Design review of the part built by this model. Coordinates are the model's own, in mm. Face numbers are marked on the shaded views. A direction names the side the tool comes from. Round coordinates to 2 decimals unless told otherwise and drop trailing zeros. Loops run counter-clockwise (first coordinate to the right, second up) from the corner with the lowest first, then second, coordinate; pieces in that order, holes last. Notation, with made-up numbers: (64, -17) -> (85, -17) arc R24 ccw to (85, 1) -> close; hole circle Ø7 at (74, -34). An arc over 180 degrees is marked (long way). Use a Markdown table: item, result. Add a question column.
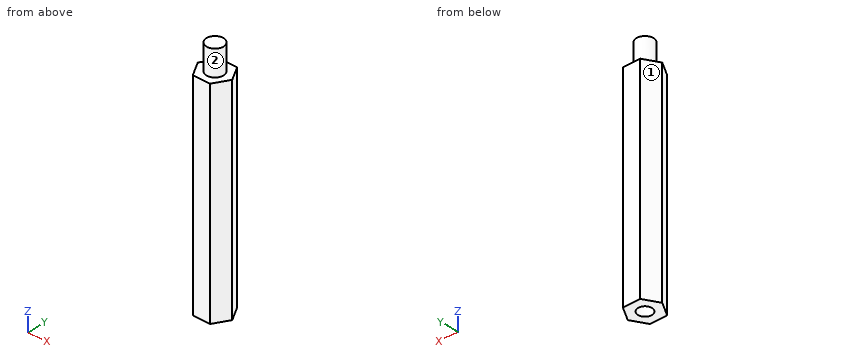
from build123d import *

# Parameters (mm, degrees)
EXTRUDE_1_DEPTH = 50
SKETCH_2_R      = 2
EXTRUDE_2_DEPTH = 6
M4X0_7_1_D      = 3.3
M4X0_7_1_DEPTH  = 10.5
M4X0_7_1_TIP    = 0.991420021


with BuildPart() as part:
    # 草圖1 → 填料-伸長1 (new body)
    with BuildSketch(Plane.XY):
        Polygon((4.041451884, 0), (2.020725942, 3.5), (-2.020725942, 3.5), (-4.041451884, 0), (-2.020725942, -3.5), (2.020725942, -3.5), align=None)
    extrude(amount=EXTRUDE_1_DEPTH)

    # 草圖2 → 填料-伸長2 (add)
    with BuildSketch(Plane.XY.offset(50)):
        Circle(SKETCH_2_R)
    extrude(amount=EXTRUDE_2_DEPTH)

    # M4x0.7 螺紋孔1
    with Locations(Plane(origin=(0, 0, 0), x_dir=(-1, 0, 0), z_dir=(0, 0, -1))):
        with Locations((0, 0)):
            Hole(M4X0_7_1_D / 2, depth=M4X0_7_1_DEPTH)
            with Locations((0, 0, -(M4X0_7_1_DEPTH + M4X0_7_1_TIP / 2))):  # 118° drill point
                Cone(0, M4X0_7_1_D / 2, M4X0_7_1_TIP, mode=Mode.SUBTRACT)


solid = part.part
1. Consider section A-A on z = 39. State the section outline as (x, y) points.
2. Insertion check: P1, Ø2, axis at x = 0, y = 0, coming from the -Z side; P2, Ø1.5, axis at y = -3, z = 44.5, coming from the -X side; P3, Ø1.5, axis at y = 2, z = 31.5, coming from the +X side; P4, Ø3, axis at x = -1, y = -2.5, coming from the -Z side. Each pin has a flat end and moves straight along its axis. Give the tip position at first contact, or say it passes through.
3. Consider section B-B on x = 2.75. State the section outline as (y, z) points.
4. Consider section C-C on y = -2.75. State the section outline as (x, z) points, plus the area to 3 significant figures.
5. To check wall thickness, follow probe 1 along Y at (x, z) = (0, 3.25); probe 2 along X at (y, z) = (0, 7.25); probe 3 along Z at (x, y) = (-0.5, 2.25). State the ranges of each line that lie inside material, in increasing order. Write a range as from..to.
6. For the marked faces 1 and 2, list the 3-axis set-ups (+Z, -Z, +X, -X, +Y, -Y) from which the entire face can be reached by the end or side of a thin tool; tool diameter is ignored.
Verdict:
| question | item | result |
|---|---|---|
| 1 | outline | (-4.04, 0) -> (-2.02, -3.5) -> (2.02, -3.5) -> (4.04, 0) -> (2.02, 3.5) -> (-2.02, 3.5) -> close |
| 2 | P1 | stops at z = 10.89 |
| 2 | P2 | stops at x = -2.74 |
| 2 | P3 | stops at x = 3.32 |
| 2 | P4 | stops at z = 0 |
| 3 | outline | (-2.24, 0) -> (2.24, 0) -> (2.24, 50) -> (-2.24, 50) -> close |
| 4 | outline | (-2.45, 0) -> (2.45, 0) -> (2.45, 50) -> (-2.45, 50) -> close |
| 4 | area | 245 mm² |
| 5 | probe 1 | y = -3.5..-1.65, 1.65..3.5 |
| 5 | probe 2 | x = -4.04..-1.65, 1.65..4.04 |
| 5 | probe 3 | z = 0..50 |
| 6 | face 1 | +Z, -Z, -X, +Y |
| 6 | face 2 | +Z |
